Could you check a few things on this model? Use its own coordinates, in mm. A direction names the side the tool comes from. Round coordinates to 2 decimals unless told otherwise and drop trailing zeros. Write each loop counter-clockwise with the first axis right and the second up, starting at its lowest first coordinate (ties: lowest second). Pieces come first, ordered by that corner, then holes. Notation, with made-up numbers: (7, -31) -> (41, -31) arc R35 cw to (41, 3) -> close; hole circle Ø9 at (-3, -20). An arc over 180 degrees is marked (long way). Answer in a Markdown table with one row per item.
from build123d import *

# Parameters (mm, degrees)
SKETCH1_W           = 50
SKETCH1_H           = 50
BOSS_EXTRUDE1_DEPTH = 5
SKETCH2_W           = 49
SKETCH2_H           = 4
CUT_EXTRUDE1_DEPTH  = 49.5
SKETCH3_R           = 0.5
CUT_EXTRUDE2_DEPTH  = 71.887234394
FILLET6_R           = 0.3


with BuildPart() as part:
    # Sketch1 → Boss-Extrude1 (new body)
    with BuildSketch(Plane(origin=(0, 0, 0), x_dir=(1, 0, 0), z_dir=(0, 1, 0))):
        with Locations((25, -25)):
            Rectangle(SKETCH1_W, SKETCH1_H)
    extrude(amount=BOSS_EXTRUDE1_DEPTH)

    # Sketch2 → Cut-Extrude1 (cut)
    with BuildSketch(Plane(origin=(0, 0, 0), x_dir=(-1, 0, 0), z_dir=(0, 0, -1))):
        with Locations((-25, 2.5)):
            Rectangle(SKETCH2_W, SKETCH2_H)
    extrude(amount=-CUT_EXTRUDE1_DEPTH, mode=Mode.SUBTRACT)

    # Sketch3 → Cut-Extrude2 (cut, through all)
    with BuildSketch(Plane(origin=(0, 5, 0), x_dir=(1, 0, 0), z_dir=(0, 1, 0))):
        with Locations(Location((24.38451422, -23.433057304, 0), (0, 0, 270))):
            Circle(SKETCH3_R)
    extrude(amount=-CUT_EXTRUDE2_DEPTH, mode=Mode.SUBTRACT)

    # Fillet6
    fillet6_edges = [part.edges().sort_by_distance(p)[0] for p in [
        (50, 5, 25),
        (49.5, 2.5, 49.5),
        (25, 5, 0),
        (49.5, 0.5, 24.75),
        (25, 4.5, 49.5),
        (49.5, 4.5, 24.75),
        (0.5, 2.5, 49.5),
        (0.5, 4.5, 24.75),
        (25, 0.5, 49.5),
        (0.5, 0.5, 24.75),
        (0, 5, 25),
        (25, 0, 0),
        (50, 0, 25),
        (25, 0, 50),
        (0, 0, 25),
        (0, 2.5, 0),
        (50, 2.5, 0),
        (50, 2.5, 50),
        (0, 2.5, 50),
        (25, 5, 50),
    ]]
    fillet(fillet6_edges, radius=FILLET6_R)


solid = part.part
1) Imagine slicing it at B-B, the plane x = 29. Please give me the cut outline in (y, z).
Findings:
| item | result |
|---|---|
| outline | (0, 0.3) arc R0.3 ccw to (0.3, 0) -> (0.5, 0) -> (0.5, 49.2) arc R0.3 cw to (0.8, 49.5) -> (4.2, 49.5) arc R0.3 cw to (4.5, 49.2) -> (4.5, 0) -> (4.7, 0) arc R0.3 ccw to (5, 0.3) -> (5, 49.7) arc R0.3 ccw to (4.7, 50) -> (0.3, 50) arc R0.3 ccw to (0, 49.7) -> close |
2) For faces 5 (the face through (50, 2, 25)), 6 (the face through (25, 4.5, 24)), which set-ups out of +Z, -Z, +X, -X, +Y, -Y let a thin tool reach every point of the face, with its end or its side?
Findings:
| item | result |
|---|---|
| face 5 | +Z, -Z, +X, +Y, -Y |
| face 6 | -Z |
3) Imagine slicing it at C-C, the plane y = 1.75. Please give me the cut outline in (x, z), plus the area to 3 significant figures.
Findings:
| item | result |
|---|---|
| outline | (0, 0.3) arc R0.3 ccw to (0.3, 0) -> (0.5, 0) -> (0.5, 49.2) arc R0.3 cw to (0.8, 49.5) -> (49.2, 49.5) arc R0.3 cw to (49.5, 49.2) -> (49.5, 0) -> (49.7, 0) arc R0.3 ccw to (50, 0.3) -> (50, 49.7) arc R0.3 ccw to (49.7, 50) -> (0.3, 50) arc R0.3 ccw to (0, 49.7) -> close |
| area | 74.5 mm^2 |
4) Imagine slicing it at A-A, the plane z = 33. Please give me the cut outline in (x, y), plus the area to 3 significant figures.
Findings:
| item | result |
|---|---|
| outline | (0, 0.3) arc R0.3 ccw to (0.3, 0) -> (49.7, 0) arc R0.3 ccw to (50, 0.3) -> (50, 4.7) arc R0.3 ccw to (49.7, 5) -> (0.3, 5) arc R0.3 ccw to (0, 4.7) -> close; hole (0.5, 0.8) arc R0.3 ccw to (0.8, 0.5) -> (49.2, 0.5) arc R0.3 ccw to (49.5, 0.8) -> (49.5, 4.2) arc R0.3 ccw to (49.2, 4.5) -> (0.8, 4.5) arc R0.3 ccw to (0.5, 4.2) -> close |
| area | 54.0 mm^2 |
5) Please list where these lines run through material, in increasing order: line 1 (X direction, y = 3.6, z = 7.5); line 2 (Y direction, x = 20.5, z = 18.5); line 3 (Z direction, x = 47, y = 1.1).
Findings:
| item | result |
|---|---|
| line 1 | x = 0 to 0.5, 49.5 to 50 |
| line 2 | y = 0 to 0.5, 4.5 to 5 |
| line 3 | z = 49.5 to 50 |
6) For pin 1 (1.7 mm diameter, centred on x = 20, y = 2, fed in from -Z), with a flat end and sliding along its axis, tell me the tip position at first contact or that it passes through.
Findings:
| item | result |
|---|---|
| pin 1 | stops at z = 49.5 |
7) Thinking about a two-plate mould opening in Y: for faces 1 (the face through (49.5, 2, 24)), 2 (the face through (25, 3, 49.5)), 3 (the face through (25, 0, 25)), 4 (the face through (25, 5, 25)), which applies, +Y half, -Y half, draft (parallel to the pull), parting line (faces both ways), or undercut?
Findings:
| item | result |
|---|---|
| face 1 | undercut |
| face 2 | undercut |
| face 3 | -Y half |
| face 4 | +Y half |
